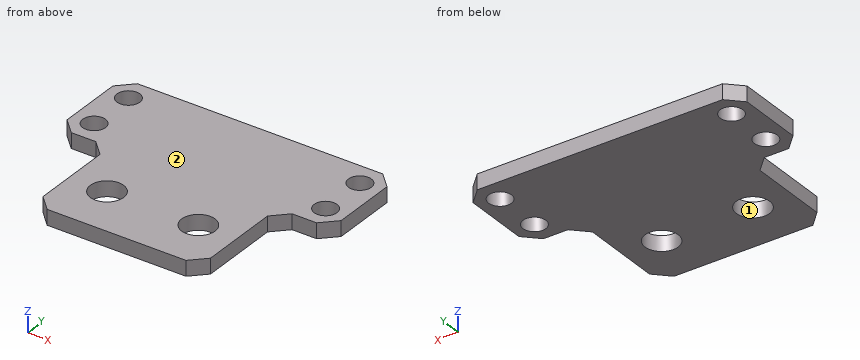
from build123d import *

# Parameters (mm, degrees)
SKETCH1_R           = 3.475
SKETCH1_R_2         = 2.3828
BOSS_EXTRUDE1_DEPTH = 3.175
CHAMFER1_SIZE       = 3
CHAMFER2_SIZE       = 3


with BuildPart() as part:
    # Sketch1 → Boss-Extrude1 (new body)
    with BuildSketch(Plane.XY):
        Polygon((17.4625, -21.209), (-17.4625, -21.209), (-17.4625, 1.651), (-28.575, 1.651), (-28.575, 21.209), (28.575, 21.209), (28.575, 1.651), (17.4625, 1.651), align=None)
        with Locations((-9.525, -10.541)):
            Circle(SKETCH1_R, mode=Mode.SUBTRACT)
        with Locations((9.525, -10.541)):
            Circle(SKETCH1_R, mode=Mode.SUBTRACT)
        with Locations((-24.13, 6.35)):
            Circle(SKETCH1_R_2, mode=Mode.SUBTRACT)
        with Locations((-24.13, 16.51)):
            Circle(SKETCH1_R_2, mode=Mode.SUBTRACT)
        with Locations((24.13, 16.51)):
            Circle(SKETCH1_R_2, mode=Mode.SUBTRACT)
        with Locations((24.13, 6.35)):
            Circle(SKETCH1_R_2, mode=Mode.SUBTRACT)
    extrude(amount=BOSS_EXTRUDE1_DEPTH)

    # Chamfer1
    chamfer1_edges = [part.edges().sort_by_distance(p)[0] for p in [
        (-28.575, 1.651, 1.5875),
        (-28.575, 21.209, 1.5875),
        (28.575, 21.209, 1.5875),
        (28.575, 1.651, 1.5875),
    ]]
    chamfer(chamfer1_edges, length=CHAMFER1_SIZE)

    # Chamfer2
    chamfer2_edges = [part.edges().sort_by_distance(p)[0] for p in [
        (17.4625, 1.651, 1.5875),
        (17.4625, -21.209, 1.5875),
        (-17.4625, -21.209, 1.5875),
        (-17.4625, 1.651, 1.5875),
    ]]
    chamfer(chamfer2_edges, length=CHAMFER2_SIZE)


solid = part.part
Input: part model. Units: mm. Frame: model coordinates. Face numbers are marked on the shaded views. Give positions to 0.01 mm unless a question says otherwise; leave off trailing zeros. Loops run counter-clockwise (first coordinate to the right, second up) from the corner with the lowest first, then second, coordinate; pieces in that order, holes last. Notation, with made-up numbers: M 32,-35.75 L 81,-35.75 A28 ccw 81,-15.75 Z; hole C 33,-6 d6. An arc over 180 degrees is marked long. Use one line per item in the form item = value.
1. First-contact query: pin 1 (1 mm diameter, centred on y = -14.5, z = 1.5, fed in from -X); pin 2 (1 mm diameter, centred on x = 24, z = 2, fed in from -Y). Flat tips, straight axial feed; report the tip coordinate or a pass-through.
Numbers:
pin_1 = -17.46
pin_2 = 1.65
2. Pull-direction query (X, two-part tool) for the marked faces 1 and 2; classes: released by +X, released by -X, zero draft, split by the parting line, or undercut.
Numbers:
face_1 = undercut
face_2 = zero draft
3. Section query D-D, the plane x = 18.5. Return the cut outline in (y, z) (1 decimal).
Numbers:
outline = M -0.3,0 L 21.2,0 L 21.2,3.2 L -0.3,3.2 Z
4. Section query C-C, the plane z = 2.25. Count the separate pieces of the cut face and the enclosed holes in it, and give its area (3 significant figures).
Numbers:
separate_pieces = 1
enclosed_holes = 6
area = 1,750 mm²
5. Section query B-B, the plane x = -24.13. Return the cut outline in (y, z) (3 decimals), and give its area (3 significant figures).
Numbers:
outline = M 1.651,0 L 3.967,0 L 3.967,3.175 L 1.651,3.175 Z; M 8.733,0 L 14.127,0 L 14.127,3.175 L 8.733,3.175 Z; M 18.893,0 L 21.209,0 L 21.209,3.175 L 18.893,3.175 Z
area = 31.8 mm²
6. Section query A-A, the plane y = 16.51. Return the cut outline in (x, z) (3 decimals), and give its area (3 significant figures).
Numbers:
outline = M -28.575,0 L -26.513,0 L -26.513,3.175 L -28.575,3.175 Z; M -21.747,0 L 21.747,0 L 21.747,3.175 L -21.747,3.175 Z; M 26.513,0 L 28.575,0 L 28.575,3.175 L 26.513,3.175 Z
area = 151 mm²
7. Line query: L1, parallel to Y at x = -24.13, z = 1.5; L2, parallel to X at y = 14.5, z = 3 (3 decimals); L3, parallel to Y at x = -23, z = 2.1. Output: solid intervals per line, ascending.
Numbers:
L1 = 1.65 to 3.97, 8.73 to 14.13, 18.89 to 21.21
L2 = -28.575 to -25.41, -22.85 to 22.85, 25.41 to 28.575
L3 = 1.65 to 4.25, 8.45 to 14.41, 18.61 to 21.21
